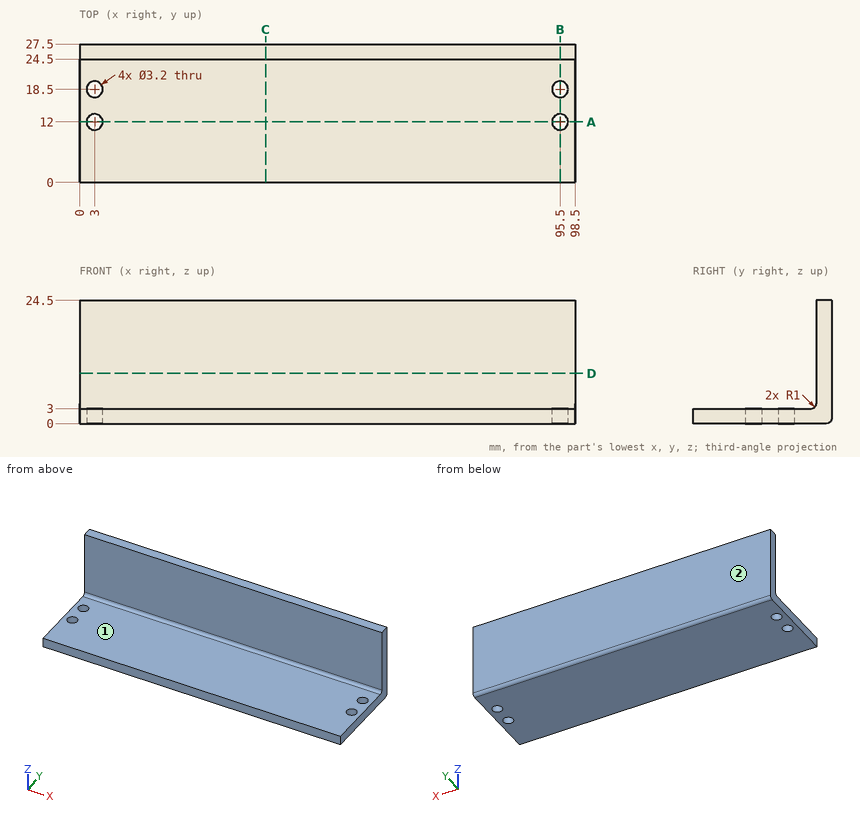
For this review, use the dimensioned drawing (mm, ordinates from the lowest corner) and the shaded views. A direction names the side the tool comes from. Round coordinates to 2 decimals unless told otherwise and drop trailing zeros. Write each loop counter-clockwise with the first axis right and the second up, starting at its lowest first coordinate (ties: lowest second). Pieces come first, ordered by that corner, then holes. Notation, with made-up numbers: (4.5, 35.5) - (34.5, 35.5) arc R28 ccw to (34.5, 68.5) - close; hole circle Ø10 at (11.25, -20.5). An arc over 180 degrees is marked (long way). One line per item, written item: value. Start each with the question number.
1. Consider section D-D on z = 10. Write out the cut boundary in (x, y).
2. Machinability: for the marked faces 1 and 2, which of the approach directions +Z, -Z, +X, -X, +Y, -Y give a long, thin tool a straight path to every point of the face, cutting with its end or side? Answer none if there is none.
3. Consider section A-A on y = 12. Write out the cut boundary in (x, z).
4. Consider section B-B on x = 95.5. Write out the cut boundary in (y, z).
5. Consider section C-C on x = 37. Write out the cut boundary in (y, z), and give its area (3 significant figures).
6. Clearance check with flat-ended pins moving along their axes: P1, Ø1, axis at x = 77.5, z = 21.5, coming from the -Y side; P2, Ø4, axis at x = 95.5, y = 18.5, coming from the -Z side; P3, Ø4, axis at x = 3, y = 12, coming from the +Z side; P4, Ø3, axis at x = 95.5, y = 12, coming from the -Z side. State where each tip first meets the part, or that it passes through.
7. To check wall thickness, follow L1, parallel to Y at x = 95.5, z = 0.9; L2, parallel to Y at x = 79.5, z = 17; L3, parallel to Z at x = 31.5, y = 21.75. State the ranges of each line that lie inside material, in increasing order. Write a range as from..to.
Checks:
1. outline: (0, 24.5) - (98.5, 24.5) - (98.5, 27.5) - (0, 27.5) - close
2. face 1: +Z, +X, -X, -Y
2. face 2: +Z, -Z, +X, -X, +Y
3. outline: (0, 0) - (1.4, 0) - (1.4, 3) - (0, 3) - close; (4.6, 0) - (93.9, 0) - (93.9, 3) - (4.6, 3) - close; (97.1, 0) - (98.5, 0) - (98.5, 3) - (97.1, 3) - close
4. outline: (0, 0) - (10.4, 0) - (10.4, 3) - (0, 3) - close; (13.6, 0) - (16.9, 0) - (16.9, 3) - (13.6, 3) - close; (20.1, 0) - (26.5, 0) arc R1 ccw to (27.5, 1) - (27.5, 24.5) - (24.5, 24.5) - (24.5, 4) arc R1 cw to (23.5, 3) - (20.1, 3) - close
5. outline: (0, 0) - (26.5, 0) arc R1 ccw to (27.5, 1) - (27.5, 24.5) - (24.5, 24.5) - (24.5, 4) arc R1 cw to (23.5, 3) - (0, 3) - close
5. area: 147 mm^2
6. P1: stops at y = 24.5
6. P2: stops at z = 0
6. P3: stops at z = 3
6. P4: passes through
7. L1: y = 0..10.4, 13.6..16.9, 20.1..27.49
7. L2: y = 24.5..27.5
7. L3: z = 0..3
